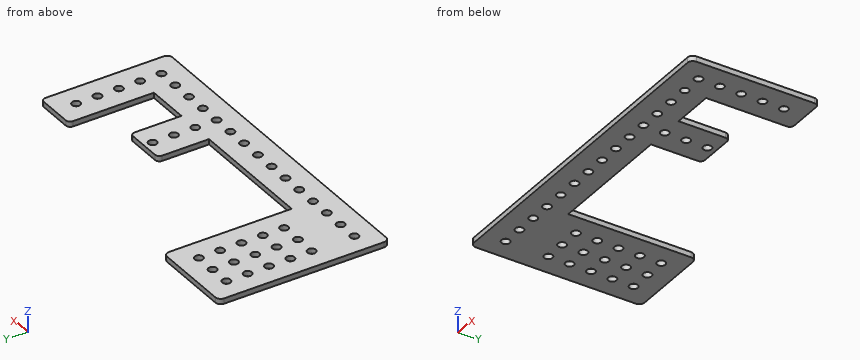
from build123d import *

# Parameters (mm, degrees)
BOSS_EXTRUDE1_DEPTH = 3.175
BOSS_EXTRUDE2_DEPTH = 3.175
SKETCH4_R           = 2.5
CUT_EXTRUDE1_DEPTH  = 4.175


with BuildPart() as part:
    # Sketch1 → Boss-Extrude1 (new body)
    with BuildSketch(Plane.XY):
        with BuildLine():
            Line((102.197610681, -20.076711723), (-50.202389319, -20.076711723))
            Line((-50.202389319, -20.076711723), (-50.202389319, 52.948288277))
            ThreePointArc((-50.202389319, 52.948288277), (-51.132325289, 55.193352307), (-53.377389319, 56.123288277))
            Line((-53.377389319, 56.123288277), (-97.827389319, 56.123288277))
            ThreePointArc((-97.827389319, 56.123288277), (-100.07245335, 55.193352307), (-101.002389319, 52.948288277))
            Line((-101.002389319, 52.948288277), (-101.002389319, -42.301711723))
            ThreePointArc((-101.002389319, -42.301711723), (-100.07245335, -44.546775753), (-97.827389319, -45.476711723))
            Line((-97.827389319, -45.476711723), (99.022610681, -45.476711723))
            ThreePointArc((99.022610681, -45.476711723), (101.267674711, -44.546775753), (102.197610681, -42.301711723))
            Line((102.197610681, -42.301711723), (102.197610681, -20.076711723))
        make_face()
    extrude(amount=BOSS_EXTRUDE1_DEPTH)

    # Sketch3 → Boss-Extrude2 (add)
    with BuildSketch(Plane.XY.offset(3.175)):
        with BuildLine():
            Line((48.857610681, 10.403288277), (28.537610681, 10.403288277))
            ThreePointArc((28.537610681, 10.403288277), (26.741559456, 9.659339501), (25.997610681, 7.863288277))
            Line((25.997610681, 7.863288277), (25.997610681, -20.076711723))
            Line((25.997610681, -20.076711723), (51.397610681, -20.076711723))
            Line((51.397610681, -20.076711723), (51.397610681, 7.863288277))
            ThreePointArc((51.397610681, 7.863288277), (50.653661905, 9.659339501), (48.857610681, 10.403288277))
        make_face()
        with BuildLine():
            Line((79.337610681, 30.723288277), (99.657610681, 30.723288277))
            ThreePointArc((99.657610681, 30.723288277), (101.453661905, 29.979339501), (102.197610681, 28.183288277))
            Line((102.197610681, 28.183288277), (102.197610681, -20.076711723))
            Line((102.197610681, -20.076711723), (76.797610681, -20.076711723))
            Line((76.797610681, -20.076711723), (76.797610681, 28.183288277))
            ThreePointArc((76.797610681, 28.183288277), (77.541559456, 29.979339501), (79.337610681, 30.723288277))
        make_face()
    extrude(amount=-BOSS_EXTRUDE2_DEPTH)

    # Sketch4 → Cut-Extrude1 (cut, through all)
    with BuildSketch(Plane.XY.offset(3.175)):
        with Locations((-88.302389319, -32.776711723)):
            Circle(SKETCH4_R)
        with Locations((-75.602389319, -32.776711723)):
            Circle(SKETCH4_R)
        with Locations((-62.902389319, -32.776711723)):
            Circle(SKETCH4_R)
        with Locations((-50.202389319, -32.776711723)):
            Circle(SKETCH4_R)
        with Locations((-37.502389319, -32.776711723)):
            Circle(SKETCH4_R)
        with Locations((-24.802389319, -32.776711723)):
            Circle(SKETCH4_R)
        with Locations((-12.102389319, -32.776711723)):
            Circle(SKETCH4_R)
        with Locations((0.597610681, -32.776711723)):
            Circle(SKETCH4_R)
        with Locations((13.297610681, -32.776711723)):
            Circle(SKETCH4_R)
        with Locations((25.997610681, -32.776711723)):
            Circle(SKETCH4_R)
        with Locations((38.697610681, -32.776711723)):
            Circle(SKETCH4_R)
        with Locations((51.397610681, -32.776711723)):
            Circle(SKETCH4_R)
        with Locations((64.097610681, -32.776711723)):
            Circle(SKETCH4_R)
        with Locations((76.797610681, -32.776711723)):
            Circle(SKETCH4_R)
        with Locations((89.497610681, -32.776711723)):
            Circle(SKETCH4_R)
        with Locations((38.697610681, -20.076711723)):
            Circle(SKETCH4_R)
        with Locations((89.497610681, -20.076711723)):
            Circle(SKETCH4_R)
        with Locations((-88.302389319, 43.423288277)):
            Circle(SKETCH4_R)
        with Locations((-62.902389319, 43.423288277)):
            Circle(SKETCH4_R)
        with Locations((-62.902389319, 30.723288277)):
            Circle(SKETCH4_R)
        with Locations((-62.902389319, 18.023288277)):
            Circle(SKETCH4_R)
        with Locations((-62.902389319, 5.323288277)):
            Circle(SKETCH4_R)
        with Locations((-62.902389319, -7.376711723)):
            Circle(SKETCH4_R)
        with Locations((-88.302389319, 30.723288277)):
            Circle(SKETCH4_R)
        with Locations((-88.302389319, 18.023288277)):
            Circle(SKETCH4_R)
        with Locations((-88.302389319, 5.323288277)):
            Circle(SKETCH4_R)
        with Locations((-88.302389319, -7.376711723)):
            Circle(SKETCH4_R)
        with Locations((38.697610681, -7.376711723)):
            Circle(SKETCH4_R)
        with Locations((89.497610681, -7.376711723)):
            Circle(SKETCH4_R)
        with Locations((38.697610681, 5.323288277)):
            Circle(SKETCH4_R)
        with Locations((89.497610681, 5.323288277)):
            Circle(SKETCH4_R)
        with Locations((89.497610681, 18.023288277)):
            Circle(SKETCH4_R)
        with Locations((-75.602389319, 43.423288277)):
            Circle(SKETCH4_R)
        with Locations((-75.602389319, 30.723288277)):
            Circle(SKETCH4_R)
        with Locations((-75.602389319, 18.023288277)):
            Circle(SKETCH4_R)
        with Locations((-75.602389319, 5.323288277)):
            Circle(SKETCH4_R)
        with Locations((-75.602389319, -7.376711723)):
            Circle(SKETCH4_R)
    extrude(amount=-CUT_EXTRUDE1_DEPTH, mode=Mode.SUBTRACT)


solid = part.part
Input: part model. Units: mm. Frame: model coordinates. Coordinates: 2 decimals unless noted, no trailing zeros. Order: outer loops, then holes, each group sorted by start corner. A loop starts at its lowest first (then second) coordinate and runs counter-clockwise, first axis right, second up. Notation, with made-up numbers: M -23,74.5 L 14,74.5 A9 cw 14,84.5 Z; hole C -12.75,0.5 d9. An arc over 180 degrees is marked long. Write item = value, one per line. Start each with the question number.
(1) Section B-B on x = -76. Output: boundary loops of the cut face in (y, z) (3 decimals), and give its area (3 significant figures).
(2) Line query: line 1 along X through (y, z) = (-20.5, 0.5); line 2 along X through (y, z) = (-20, 2.15); line 3 along X through (y, z) = (-11, 3.05). Output: solid intervals per line, ascending. Write a range as [from, to].
(3) First-contact query: P1, Ø4.5, axis at x = -24.8, y = -32.78, coming from the -Z side; P2, Ø6.5, axis at x = -62.9, y = 30.72, coming from the -Z side; P3, Ø1, axis at y = 40, z = 0.5, coming from the +X side. Flat tips, straight axial feed; report the tip coordinate or a pass-through.
(4) Section D-D on y = 37. Output: boundary loops of the cut face in (x, z) (3 decimals).
(5) Section C-C on z = 2.2. Give the number of separate pieces and of enclosed holes in the cut face, and give its area (3 significant figures).
(6) Section A-A on y = -14. Output: boundary loops of the cut face in (x, z) (3 decimals), and give its area (3 significant figures).
Result set:
q1.outline = M -45.477,0 L -35.245,0 L -35.245,3.175 L -45.477,3.175 Z; M -30.309,0 L -9.845,0 L -9.845,3.175 L -30.309,3.175 Z; M -4.909,0 L 2.855,0 L 2.855,3.175 L -4.909,3.175 Z; M 7.791,0 L 15.555,0 L 15.555,3.175 L 7.791,3.175 Z; M 20.491,0 L 28.255,0 L 28.255,3.175 L 20.491,3.175 Z; M 33.191,0 L 40.955,0 L 40.955,3.175 L 33.191,3.175 Z; M 45.891,0 L 56.123,0 L 56.123,3.175 L 45.891,3.175 Z
q1.area = 229 mm²
q2.line_1 = [-101, 36.23], [41.16, 87.03], [91.96, 102.2]
q2.line_2 = [-101, -50.2], [26, 36.2], [41.2, 51.4], [76.8, 87], [92, 102.2]
q2.line_3 = [-101, -50.2], [26, 51.4], [76.8, 102.2]
q3.P1 = through
q3.P2 = 0
q3.P3 = -50.2
q4.outline = M -101.002,0 L -50.202,0 L -50.202,3.175 L -101.002,3.175 Z
q5.separate_pieces = 1
q5.enclosed_holes = 37
q5.area = 10,400 mm²
q6.outline = M -101.002,0 L -50.202,0 L -50.202,3.175 L -101.002,3.175 Z; M 25.998,0 L 51.398,0 L 51.398,3.175 L 25.998,3.175 Z; M 76.798,0 L 102.198,0 L 102.198,3.175 L 76.798,3.175 Z
q6.area = 323 mm²
